The model under review builds one solid part; all positions refer to its coordinate system, in mm. A direction names the side the tool comes from. Give positions to 0.01 mm unless a question says otherwise; leave off trailing zeros. Write each loop counter-clockwise with the first axis right and the second up, starting at its lowest first coordinate (ties: lowest second). Pieces come first, ordered by that corner, then holes. Notation, with made-up numbers: (-33, -22) - (-20, -22) arc R21 cw to (-20, 17) - close; hole circle Ø10 at (35, 49.25). An arc over 180 degrees is marked (long way). One line per question, with ' | ' between items. Start each with the question number.
```python
from build123d import *

# Parameters (mm, degrees)
F1_DEPTH = 8.128
F0_W     = 11.684
F0_H     = 65.8876
F2_DEPTH = 25.4


with BuildPart() as f1:
    # F0 (on Top) → F1 (new body)
    with BuildSketch(Plane.XY):
        Polygon((18.796, -32.9438), (18.796, 32.9438), (1.651, 32.9438), (1.651, 32.1818), (-1.651, 32.1818), (-1.651, 32.9438), (-18.796, 32.9438), (-18.796, -32.9438), (-11.049, -32.9438), (-11.049, -32.1818), (-7.747, -32.1818), (-7.747, -32.9438), (7.747, -32.9438), (7.747, -32.1818), (11.049, -32.1818), (11.049, -32.9438), align=None)
    extrude(amount=F1_DEPTH)

    # F0 (on Top) → F2 (join)
    with BuildSketch(Plane.XY):
        with Locations((-24.638, 0)):
            Rectangle(F0_W, F0_H)
        with Locations((24.638, 0)):
            Rectangle(F0_W, F0_H)
    extrude(amount=F2_DEPTH)


solid = f1.part
```
Item 1: Take a section at C-C (x = -14.5). Give the boundary of the cut face in (y, z), plus the area to 3 significant figures.
Item 2: Machinability: for faces 1 (the flat face through (0, -32.944, 4)), 2 (the flat face through (19, 32.944, 10)), 3 (the flat face through (0, 0, 8.128)), 4 (the flat face through (0, 32.182, 4)), 5 (the flat face through (9, -32.182, 4)), which of the approach directions +Z, -Z, +X, -X, +Y, -Y give a long, thin tool a straight path to every point of the face, cutting with its end or side? Answer none if there is none.
Item 3: The part is to be moulded in two halves that separate along X. For faces 6 (the flat face through (30.48, 0, 13)), 7 (the flat face through (23, -32.944, 10)), 8 (the flat face through (-9, -32.182, 4)), say which applies: +X half, -X half, draft (parallel to the pull), parting line (faces both ways), or undercut.
Item 4: Clearance check with flat-ended pins moving along their axes: P1, Ø2, axis at x = -12.5, y = 21, coming from the +Z side; P2, Ø3.5, axis at x = -8.5, z = 6, coming from the -Y side; P3, Ø1.7, axis at x = 0, z = 5.5, coming from the +Y side. State where each tip first meets the part, or that it passes through.
Item 5: For probe 1 along X at (y, z) = (4, 23.5); probe 2 along Z at (x, y) = (0.5, -26); probe 3 along Y at (x, z) = (10, 6.25), list the stretches that pass through material, from the lowest coordinate up.
Item 6: Take a section at B-B (y = -9). Give the boundary of the cut face in (x, z), plus the area to 3 significant figures.
Item 7: Take a section at A-A (z = 12.25). Give the boundary of the cut face in (x, y), plus the area to 3 significant figures.
Check sheet entries:
1) outline: (-32.94, 0) - (32.94, 0) - (32.94, 8.13) - (-32.94, 8.13) - close | area: 536 mm^2
2) face 1: +Z, -Z, +X, -X, -Y | face 2: +Z, -Z, +X, -X, +Y | face 3: +Z, +Y, -Y | face 4: +Z, -Z, +Y | face 5: +Z, -Z, -Y
3) face 6: +X half | face 7: draft | face 8: undercut
4) P1: stops at z = 8.13 | P2: stops at y = -32.94 | P3: stops at y = 32.18
5) probe 1: x = -30.48 to -18.8, 18.8 to 30.48 | probe 2: z = 0 to 8.13 | probe 3: y = -32.18 to 32.94
6) outline: (-30.48, 0) - (30.48, 0) - (30.48, 25.4) - (18.8, 25.4) - (18.8, 8.13) - (-18.8, 8.13) - (-18.8, 25.4) - (-30.48, 25.4) - close | area: 899 mm^2
7) outline: (-30.48, -32.94) - (-18.8, -32.94) - (-18.8, 32.94) - (-30.48, 32.94) - close; (18.8, -32.94) - (30.48, -32.94) - (30.48, 32.94) - (18.8, 32.94) - close | area: 1,540 mm^2
